Could you check a few things on this model? Use its own coordinates, in mm. A direction names the side the tool comes from. Coordinates: 2 decimals unless noted, no trailing zeros. Loops run counter-clockwise (first coordinate to the right, second up) from the corner with the lowest first, then second, coordinate; pieces in that order, holes last. Notation, with made-up numbers: (20, 86.25) -> (77, 86.25) arc R16 cw to (77, 108.25) -> close; hole circle Ø3 at (-2.75, 59.5). An arc over 180 degrees is marked (long way). One line per question, with ' | ' between items.
from build123d import *

# Parameters (mm, degrees)
SKETCH_1_R          = 16
SKETCH_1_R_2        = 1.95
EXTRUDE_1_DEPTH     = 3
CUT_EXTRUDE_1_DEPTH = 56.599010783
FILLET_1_R          = 2


with BuildPart() as part:
    # 草图1 → 凸台-拉伸1 (new body)
    with BuildSketch(Plane.XY):
        with BuildLine():
            Line((-40, -28.5), (-40, -38.5))
            Line((-40, -38.5), (40, -38.5))
            Line((40, -38.5), (40, -28.5))
            Line((40, -28.5), (18.328389928, 10.250371829))
            ThreePointArc((18.328389928, 10.250371829), (0, 21), (-18.328389928, 10.250371829))
            Line((-18.328389928, 10.250371829), (-40, -28.5))
        make_face()
        Circle(SKETCH_1_R, mode=Mode.SUBTRACT)
        with Locations((27, -33.5)):
            Circle(SKETCH_1_R_2, mode=Mode.SUBTRACT)
        with Locations((19, -33.5)):
            Circle(SKETCH_1_R_2, mode=Mode.SUBTRACT)
        with Locations((-27, -33.5)):
            Circle(SKETCH_1_R_2, mode=Mode.SUBTRACT)
        with Locations((-19, -33.5)):
            Circle(SKETCH_1_R_2, mode=Mode.SUBTRACT)
    extrude(amount=EXTRUDE_1_DEPTH)

    # 草图2 → 切除-拉伸1 (cut, through all)
    with BuildSketch(Plane.XY.offset(3)):
        with BuildLine():
            Line((-31.979655574, -28.5), (-5, -28.5))
            Line((-5, -28.5), (-5, -20.396078054))
            ThreePointArc((-5, -20.396078054), (-14.160497384, -15.507427699), (-19.859102687, -6.827594046))
            Line((-19.859102687, -6.827594046), (-31.979655574, -28.5))
        make_face()
        with BuildLine():
            Line((19.859102687, -6.827594046), (31.979655574, -28.5))
            Line((31.979655574, -28.5), (5, -28.5))
            Line((5, -28.5), (5, -20.396078054))
            ThreePointArc((5, -20.396078054), (14.160497384, -15.507427699), (19.859102687, -6.827594046))
        make_face()
    extrude(amount=-CUT_EXTRUDE_1_DEPTH, mode=Mode.SUBTRACT)

    # 圆角1
    fillet_1_edges = [part.edges().sort_by_distance(p)[0] for p in [
        (40, -28.5, 1.5),
        (40, -38.5, 1.5),
        (-40, -38.5, 1.5),
        (-40, -28.5, 1.5),
        (5, -20.396078054, 1.5),
        (19.859102687, -6.827594046, 1.5),
        (31.979655574, -28.5, 1.5),
        (5, -28.5, 1.5),
        (-31.979655574, -28.5, 1.5),
        (-19.859102687, -6.827594046, 1.5),
        (-5, -20.396078054, 1.5),
        (-5, -28.5, 1.5),
    ]]
    fillet(fillet_1_edges, radius=FILLET_1_R)


solid = part.part
1) I need wall thicknesses on line 1 along Y through (x, z) = (0, 2.1); line 2 along X through (y, z) = (-33, 1); line 3 along Y through (x, z) = (27, 1.5). Which ranges of each line are inside material? Lowest first, please. Write a range as from..to.
Data:
line 1: -38.5..-16, 16..21 | line 2: -40..-28.88, -25.12..-20.88, -17.12..17.12, 20.88..25.12, 28.88..40 | line 3: -38.5..-35.45, -31.55..-28.5, -19.6..-5.26
2) If we section it at B-B on y = 0: Please give me the cut outline in (x, z).
Data:
outline: (-24.06, 0) -> (-16, 0) -> (-16, 3) -> (-24.06, 3) -> close; (16, 0) -> (24.06, 0) -> (24.06, 3) -> (16, 3) -> close
3) On a 3-axis mill with a long thin cutter (end or side, diameter ignored), from which of +Z, -Z, +X, -X, +Y, -Y can I reach the whole of each face in a straight line? I mean faces 1 (the face through (29.19, -9.17, 1.48)), 2 (the face through (13.18, -16.35, 1.52)). Say none if no direction works.
Data:
face 1: +Z, -Z, +X, +Y | face 2: +Z, -Z
4) I'm going to push flat-ended pins straight in: pin 1 Ø1.5 at (y, z) = (1, 1.5) entering from -X; pin 2 Ø1.5 at (x, z) = (-18, 1.5) entering from +Y; pin 3 Ø0.9 at (y, z) = (-24, 1) entering from -X (3 decimals). Where does each tip first touch, or does it pass through?
Data:
pin 1: x = -23.92 | pin 2: y = 11.98 | pin 3: x = -37.735
5) If we section it at C-C on z = 1.15: Give the number of separate pieces and of enclosed holes in the cut face, and give its area (3 significant figures).
Data:
separate pieces: 1 | enclosed holes: 7 | area: 1,870 mm²
6) If we section it at D-D on x = 27: Please give me the cut outline in (y, z).
Data:
outline: (-38.5, 0) -> (-35.45, 0) -> (-35.45, 3) -> (-38.5, 3) -> close; (-31.55, 0) -> (-28.5, 0) -> (-28.5, 3) -> (-31.55, 3) -> close; (-19.6, 0) -> (-5.26, 0) -> (-5.26, 3) -> (-19.6, 3) -> close
7) If we section it at A-A on x = 0: Please give me the cut outline in (y, z), and give its area (3 significant figures).
Data:
outline: (-38.5, 0) -> (-16, 0) -> (-16, 3) -> (-38.5, 3) -> close; (16, 0) -> (21, 0) -> (21, 3) -> (16, 3) -> close | area: 82.5 mm²
8) We'd pull the mould along Y, two halves only. Please class faces 3 (the face through (18, -28.5, 2)), 4 (the face through (17.052, -33.414, 1.479)), 5 (the face through (-28.887, -8.629, 1.479)), 6 (the face through (-39.43, -37.9, 1.52)): pulls with the +Y half, pulls with the -Y half, needs draft (parallel to the pull), parting line crosses it, or undercut.
Data:
face 3: undercut | face 4: undercut | face 5: pulls with the +Y half | face 6: pulls with the -Y half
